from build123d import *

# Parameters (mm, degrees)
SKETCH1_R           = 50
BOSS_EXTRUDE2_DEPTH = 15
SHELL1_T            = -4
SKETCH3_R           = 27.405
BOSS_EXTRUDE3_DEPTH = 4


with BuildPart() as part:
    # Sketch1 → Boss-Extrude2 (new body)
    with BuildSketch(Plane(origin=(0, 0, 0), x_dir=(1, 0, 0), z_dir=(0, 1, 0))):
        with Locations(Location((0, 0, 0), (0, 0, 270))):
            Circle(SKETCH1_R)
    extrude(amount=BOSS_EXTRUDE2_DEPTH)

    # Shell1
    shell1_openings = [part.faces().sort_by_distance(p)[0] for p in [
        (0, 15, 0),
    ]]
    offset(amount=SHELL1_T, openings=shell1_openings, kind=Kind.INTERSECTION)

    # Sketch3 → Boss-Extrude3 (add)
    with BuildSketch(Plane(origin=(0, 4, 0), x_dir=(1, 0, 0), z_dir=(0, 1, 0))):
        with Locations(Location((0, 0, 0), (0, 0, 270))):
            Circle(SKETCH3_R)
    extrude(amount=BOSS_EXTRUDE3_DEPTH)


solid = part.part
Read the model definition and answer for the solid it produces. Units are mm, in the model's axes. A direction names the side the tool comes from. Give positions to 0.01 mm unless a question says otherwise; leave off trailing zeros. Write each loop counter-clockwise with the first axis right and the second up, starting at its lowest first coordinate (ties: lowest second). Pieces come first, ordered by that corner, then holes. Notation, with made-up numbers: (-29, -33) - (-22, -33) arc R26 cw to (-22, 4) - close; hole circle Ø5 at (88, -20). An arc over 180 degrees is marked (long way). Return JSON: item names as keys, results as strings.
Q1. A cutting plane is placed at B-B, the plane z = 0. Determine the outline of the cut face in (x, y) (3 decimals).
Reply:
{"outline": "(-50, 0) - (50, 0) - (50, 15) - (46, 15) - (46, 4) - (27.405, 4) - (27.405, 8) - (-27.405, 8) - (-27.405, 4) - (-46, 4) - (-46, 15) - (-50, 15) - close"}
Q2. For faces 1 (the face through (0, 8, 0)), 2 (the face through (1, 0, -1)), determine the directions among +Z, -Z, +X, -X, +Y, -Y from which every point of the face is accessible in a straight line to the end or side of a thin tool.
Reply:
{"face 1": "+Y", "face 2": "+Z, -Z, +X, -X, -Y"}
Q3. Given P1, Ø5, axis at x = -18.5, z = 29, coming from the -Y side; P2, Ø1.5, axis at y = 8.5, z = -6, coming from the +X side; P3, Ø6, axis at y = 1.5, z = 2.5, coming from the -X side; P4, Ø1.5, axis at y = 10.5, z = -24.5, coming from the -X side, each flat-ended and moving along its own axis, determine where each tip first touches the part or whether it passes through.
Reply:
{"P1": "y = 0", "P2": "x = 49.72", "P3": "x = -50", "P4": "x = -44"}
Q4. For a pull along Z with two mould halves and no side action, classify faces 3 (the face through (-41, 15, 22)), 4 (the face through (-20, 4, 20)), 5 (the face through (15.02, 7.4, 47.69)) as released by +Z, released by -Z, zero draft, split by the parting line, or undercut.
Reply:
{"face 3": "zero draft", "face 4": "undercut", "face 5": "split by the parting line"}
Q5. A cutting plane is placed at C-C, the plane y = 13. Determine the outline of the cut face in (x, z), and give its area (3 significant figures).
Reply:
{"outline": "circle Ø100 at (0, 0); hole circle Ø92 at (0, 0)", "area": "1,210 mm²"}
Q6. Consider line 1 along X through (y, z) = (7.5, -23); line 2 along X through (y, z) = (6, -3); line 3 along Z through (x, y) = (22, 6). Determine where each line is inside the solid, lowest interval first. Write a range as [from, to].
Reply:
{"line 1": "[-44.4, -39.84], [-14.9, 14.9], [39.84, 44.4]", "line 2": "[-49.91, -45.9], [-27.24, 27.24], [45.9, 49.91]", "line 3": "[-44.9, -40.4], [-16.34, 16.34], [40.4, 44.9]"}
Q7. A cutting plane is placed at D-D, the plane y = 2.75. Determine the outline of the cut face in (x, z).
Reply:
{"outline": "circle Ø100 at (0, 0)"}
Q8. A cutting plane is placed at A-A, the plane x = 0. Determine the outline of the cut face in (y, z) (3 decimals).
Reply:
{"outline": "(0, -50) - (15, -50) - (15, -46) - (4, -46) - (4, -27.405) - (8, -27.405) - (8, 27.405) - (4, 27.405) - (4, 46) - (15, 46) - (15, 50) - (0, 50) - close"}
